Source: CAD feature listing. Evaluate the final solid. Frame: model axes, mm. Give positions to 0.01 mm unless a question says otherwise; leave off trailing zeros. Loops run counter-clockwise (first coordinate to the right, second up) from the corner with the lowest first, then second, coordinate; pieces in that order, holes last. Notation, with made-up numbers: (26.25, 29) - (74.25, 29) arc R27 cw to (74.25, 64) - close; hole circle Ø2 at (83.5, -30). An arc over 180 degrees is marked (long way). Put each result on its own line as item: value.
```python
from build123d import *

# Parameters (mm, degrees)
SKETCH1_W          = 12
SKETCH1_H          = 12
EXTRUDE1_DEPTH     = 150
SKETCH2_W          = 5
SKETCH2_H          = 1
CUT_EXTRUDE2_DEPTH = 151.956947505
CUT_EXTRUDE3_DEPTH = 151.956947505
CUT_EXTRUDE4_DEPTH = 151.956947505
CUT_EXTRUDE5_DEPTH = 151.956947505


with BuildPart() as part:
    # Sketch1 → Extrude1 (new body)
    with BuildSketch(Plane.XY):
        with Locations((6, 6)):
            Rectangle(SKETCH1_W, SKETCH1_H)
    extrude(amount=EXTRUDE1_DEPTH)

    # Sketch2 → Cut-Extrude2 (cut, through all)
    with BuildSketch(Plane(origin=(12, 0, 0), x_dir=(0, 0, -1), z_dir=(1, 0, 0))):
        with Locations((-2.5, 0.5)):
            Rectangle(SKETCH2_W, SKETCH2_H)
        with Locations((-147.5, 0.5)):
            Rectangle(SKETCH2_W, SKETCH2_H)
    extrude(amount=-CUT_EXTRUDE2_DEPTH, mode=Mode.SUBTRACT)

    # Sketch3 → Cut-Extrude3 (cut, through all)
    with BuildSketch(Plane(origin=(12, 0, 0), x_dir=(0, 0, -1), z_dir=(1, 0, 0))):
        Polygon((-150, 2.7), (-145, 2.7), (-144.383716857, 5), (-139, 5), (-137.124355653, 12), (-150, 12), align=None)
        Polygon((0, 2.7), (-5, 2.7), (-5.616283143, 5), (-11, 5), (-12.875644347, 12), (0, 12), align=None)
    extrude(amount=-CUT_EXTRUDE3_DEPTH, mode=Mode.SUBTRACT)

    # Sketch4 → Cut-Extrude4 (cut, through all)
    with BuildSketch(Plane(origin=(12, 0, 0), x_dir=(0, 0, -1), z_dir=(1, 0, 0))):
        Polygon((-145, 1), (-145, 1.087275325), (-150, 1), align=None)
        Polygon((-145, 2.7), (-145, 2.612724675), (-150, 2.7), align=None)
        Polygon((-5, 2.7), (-5, 2.612724675), (0, 2.7), align=None)
        Polygon((-5, 1), (-5, 1.087275325), (0, 1), align=None)
    extrude(amount=-CUT_EXTRUDE4_DEPTH, mode=Mode.SUBTRACT)

    # Sketch5 → Cut-Extrude5 (cut, through all)
    with BuildSketch(Plane(origin=(12, 0, 0), x_dir=(0, 0, -1), z_dir=(1, 0, 0))):
        Polygon((-149.851496055, 1.002592146), (-150, 2.7), (-150, 1), align=None)
        with BuildLine():
            Line((-145, 2.612724675), (-150, 2.7))
            Line((-150, 2.7), (-147.05511845, 2.127573014))
            ThreePointArc((-147.05511845, 2.127573014), (-146.011481885, 2.302044703), (-145, 2.612724675))
        make_face()
        Polygon((0, 1), (0, 2.7), (-0.148503945, 1.002592146), align=None)
    extrude(amount=-CUT_EXTRUDE5_DEPTH, mode=Mode.SUBTRACT)


solid = part.part
```
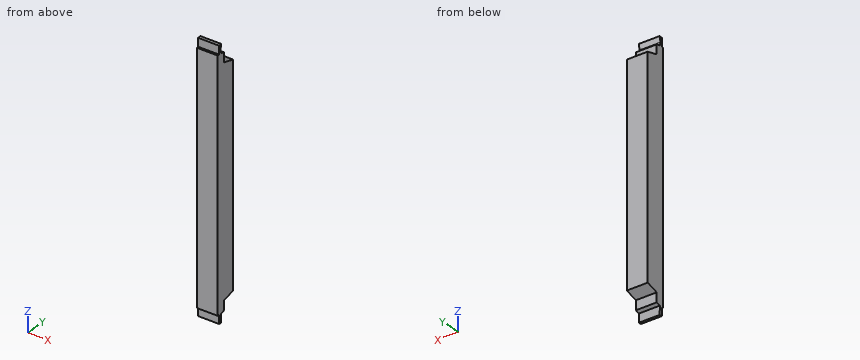
1) Section query A-A, the plane x = 7.5. Output: boundary loops of the cut face in (y, z), plus the area to 3 significant figures.
Check result:
outline: (0, 5) - (1.09, 5) - (1, 0.15) - (2.7, 0) - (2.61, 5) - (2.7, 5) - (5, 5.62) - (5, 11) - (12, 12.88) - (12, 137.12) - (5, 139) - (5, 144.38) - (2.7, 145) - (2.61, 145) arc R8 cw to (2.13, 147.06) - (2.7, 150) - (1, 149.85) - (1.09, 145) - (0, 145) - close
area: 1,600 mm²
2) Section query B-B, the plane y = 8.5. Output: boundary loops of the cut face in (x, z), plus the area to 3 significant figures.
Check result:
outline: (0, 11.94) - (12, 11.94) - (12, 138.06) - (0, 138.06) - close
area: 1,510 mm²
3) Material intervals for line 1 along Y through (x, z) = (6, 140); line 2 along Z through (x, y) = (1.25, 6.75); line 3 along Z through (x, y) = (3.25, 7.25), sorted ascending. Write a range as [from, to].
Check result:
line 1: [0, 5]
line 2: [11.47, 138.53]
line 3: [11.6, 138.4]
4) Pin query (flat end, axial travel): P1, Ø4, axis at x = 8.5, y = 7.5, coming from the +Z side; P2, Ø2.5, axis at x = 5, z = 9.5, coming from the +Y side; P3, Ø0.9, axis at x = 8, y = 0.5, coming from the +Z side; P4, Ø5, axis at y = 5, z = 106, coming from the -X side. Return the tip coordinate at first contact, or that it passes through.
Check result:
P1: z = 138.87
P2: y = 5
P3: z = 145
P4: x = 0
